Study the drawing (mm; zero at the part's minimum x, y, z) and answer. Round coordinates to 2 decimals unless told otherwise and drop trailing zeros. Order: outer loops, then holes, each group sorted by start corner. A loop starts at its lowest first (then second) coordinate and runs counter-clockwise, first axis right, second up. Notation, with made-up numbers: M 73,42.25 L 94,42.25 A35 ccw 94,81.25 Z; hole C -28,81.5 d4. An arc over 180 degrees is marked long. Put each result on its own line as item: value. Start each with the question number.
1. The part is cut by section B-B (y = 14.75). Give the vertices of the cut face in (x, z).
2. The part is cut by section D-D (x = 83). Give the vertices of the cut face in (y, z).
3. Consider line 1 (Z direction, x = 529, y = 22.5); line 2 (X direction, y = 21, z = 54.5); line 3 (X direction, y = 21, z = 140.5). Determine where each line is inside the solid, lowest interval first.
4. The part is cut by section A-A (x = 961). Give the vertices of the cut face in (y, z).
5. Each of these flat-tipped pins is pushed along its axis until it touches: pin 1 Ø15 at (x, y) = (1155.5, 21) entering from -Z; pin 2 Ø15 at (x, y) = (1159, 13.5) entering from +Z. Where does it stop, or does it pass through?
6. The part is cut by section C-C (z = 125). Give the vertices of the cut face in (x, y), then the cut area to 3 significant figures.
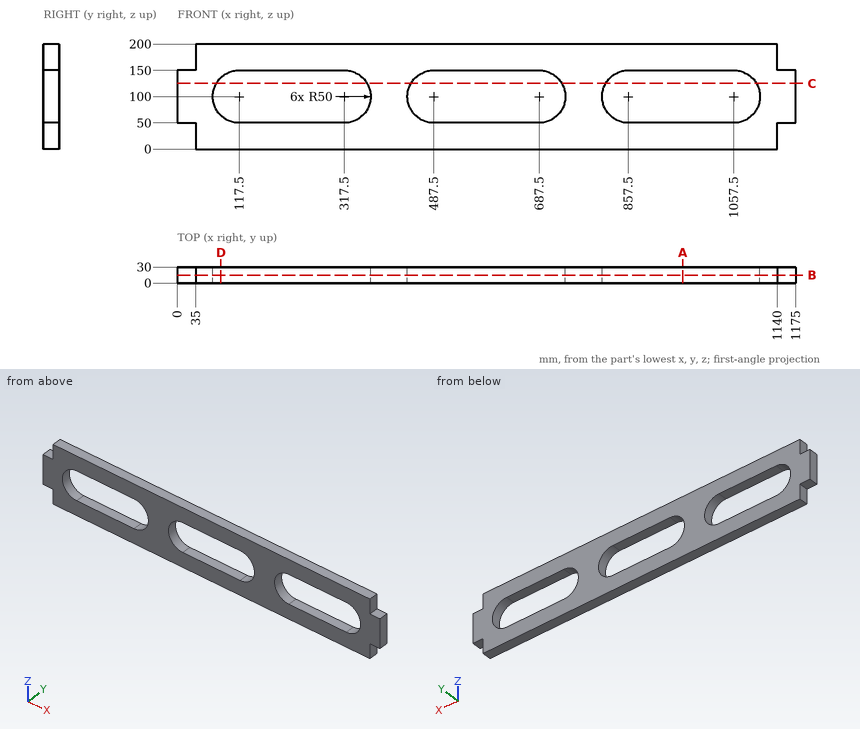
Resolved:
1. outline: M 0,50 L 35,50 L 35,0 L 1140,0 L 1140,50 L 1175,50 L 1175,150 L 1140,150 L 1140,200 L 35,200 L 35,150 L 0,150 Z; hole M 117.5,50 L 317.5,50 A50 ccw 317.5,150 L 117.5,150 A50 ccw Z; hole M 487.5,50 L 687.5,50 A50 ccw 687.5,150 L 487.5,150 A50 ccw Z; hole M 857.5,50 L 1057.5,50 A50 ccw 1057.5,150 L 857.5,150 A50 ccw Z
2. outline: M 0,0 L 30,0 L 30,63.81 L 0,63.81 Z; M 0,136.19 L 30,136.19 L 30,200 L 0,200 Z
3. line 1: 0 to 50, 150 to 200
3. line 2: 0 to 96.77, 338.23 to 466.77, 708.23 to 836.77, 1078.23 to 1175
3. line 3: 0 to 88.18, 346.82 to 458.18, 716.82 to 828.18, 1086.82 to 1175
4. outline: M 0,0 L 30,0 L 30,50 L 0,50 Z; M 0,150 L 30,150 L 30,200 L 0,200 Z
5. pin 1: z = 50
5. pin 2: z = 150
6. outline: M 0,0 L 74.2,0 L 74.2,30 L 0,30 Z; M 360.8,0 L 444.2,0 L 444.2,30 L 360.8,30 Z; M 730.8,0 L 814.2,0 L 814.2,30 L 730.8,30 Z; M 1100.8,0 L 1175,0 L 1175,30 L 1100.8,30 Z
6. area: 9,460 mm2
